Autodesk Fusion 360 part; units mm, degrees
sketch "Sketch1" plane through (0, 0, 0) normal (0, 0, 1) x (1, 0, 0)
  line L0 (30.2, 81.2805) -> (41.5, 81.2805)
  line L1 (41.5, 81.2805) -> (41.5, -5.4195)
  line L2 (41.5, -5.4195) -> (30.2, -5.4195)
  line L3 (30.2, -5.4195) -> (30.2, 81.2805)
  circle A0 centre (36.5, 3.0805) radius 1.5
  circle A1 centre (35.2, 72.7805) radius 1.5
  dimension "d1" = 1.3
  dimension "d2" = 69.7
  dimension "d3" = 3
  dimension "d4" = 3
  dimension "d5" = 5
  dimension "d6" = 5
  dimension "d7" = 8.5
  dimension "d8" = 8.5
extrude "Extrude1" add sketch "Sketch1" along normal blind 3
sketch "Sketch2" plane through (0, 0, 3) normal (0, 0, 1) x (-1, 0, 0)
  circle A0 centre (-36.5, -3.0805) radius 1.5
  circle A1 centre (-35.2, -72.7805) radius 1.5
  line L0 (-30.2, 5.4195) -> (-41.5, 5.4195)
  line L1 (-41.5, 5.4195) -> (-41.5, -81.2805)
  line L2 (-41.5, -81.2805) -> (-30.2, -81.2805)
  line L3 (-30.2, -81.2805) -> (-30.2, 5.4195)
  line L4 (-30.2, -53.1183) -> (-41.5, -53.1183)
  line L5 (-41.5, -53.1183) -> (-41.5, -31.956)
  line L6 (-41.5, -31.956) -> (-30.2, -31.956)
  line L7 (-30.2, -31.956) -> (-30.2, -53.1183)
extrude "Extrude2" add sketch "Sketch2" along normal blind 38.1 contours L1 L3 L4 L5 L6 L7
sketch "Sketch3" plane through (41.5, 0, 0) normal (1, 0, 0) x (0, 1, 0)
  line L0 (-5.4195, 0) -> (81.2805, 0)
  line L1 (81.2805, 0) -> (81.2805, 3)
  line L2 (81.2805, 3) -> (53.1183, 3)
  line L3 (53.1183, 3) -> (53.1183, 41.1)
  line L4 (53.1183, 41.1) -> (31.956, 41.1)
  line L5 (31.956, 41.1) -> (31.956, 3)
  line L6 (31.956, 3) -> (-5.4195, 3)
  line L7 (-5.4195, 3) -> (-5.4195, 0)
  line L8 (31.956, 34.75) -> (47, 34.75)
  line L9 (47, 34.75) -> (47, 31.575)
  line L10 (47, 31.575) -> (31.956, 31.575)
  line L11 (31.956, 31.575) -> (31.956, 34.75)
  line L12 (31.956, 12.525) -> (47, 12.525)
  line L13 (47, 12.525) -> (47, 9.35)
  line L14 (47, 9.35) -> (31.956, 9.35)
  line L15 (31.956, 9.35) -> (31.956, 12.525)
  dimension "d13" = 3.175
  dimension "d14" = 3.175
  dimension "d15" = 19.05
  dimension "d16" = 6.35
extrude "Extrude3" cut sketch "Sketch3" against normal blind 15 contours L5 L12 L13 L14 L15 | L5 L8 L9 L10 L11
sketch "Sketch4" plane through (0, 0, 41.1) normal (0, 0, 1) x (-1, 0, 0)
  line L0 (-30.2, -31.956) -> (-41.5, -31.956)
  line L1 (-41.5, -31.956) -> (-41.5, -53.1183)
  line L2 (-41.5, -53.1183) -> (-30.2, -53.1183)
  line L3 (-30.2, -53.1183) -> (-30.2, -31.956)
  circle A0 centre (-35.85, -34.956) radius 1.5
  circle A1 centre (-35.85, -42.956) radius 1.5
  dimension "d19" = 3
  dimension "d20" = 3
  dimension "d21" = 3
  dimension "d22" = 8
extrude "Extrude4" cut sketch "Sketch4" against normal blind 30 contours A0 | A1
Verification items for the finished model (mm, model axes). A direction names the side the tool comes from. Give positions to 0.01 mm unless a question says otherwise; leave off trailing zeros. Order: outer loops, then holes, each group sorted by start corner. A loop starts at its lowest first (then second) coordinate and runs counter-clockwise, first axis right, second up. Notation, with made-up numbers: (51.25, 37.5) -> (103.25, 37.5) arc R24 cw to (103.25, 48.5) -> close; hole circle Ø9 at (65.25, 60). An arc over 180 degrees is marked (long way). One line per item, written item: value.
(1) Tool access check on faces 1 (the face through (36, 31.956, 22)), 2 (the face through (41.5, 41, 16)), 3 (the face through (35.16, 36.29, 37.97)), 4 (the face through (36, 40, 9.35)). Record the directions out of +Z, -Z, +X, -X, +Y, -Y that give a thin tool (end or side, any length) a straight path to the whole face; none if there is none.
Final values:
face 1: +Z, +X, -X, -Y
face 2: +Z, -Z, +X, +Y, -Y
face 3: +Z
face 4: +X, -X, -Y
(2) Scan lines: line 1 along Y through (x, z) = (35.85, 19); line 2 along Z through (x, y) = (40, 38) (3 decimals); line 3 along Y through (x, z) = (36.5, 0.7). Record each from-to range of solid material in increasing order. Write a range as [from, to].
Final values:
line 1: [31.96, 33.46], [36.46, 41.46], [44.46, 53.12]
line 2: [0, 9.35], [12.525, 31.575], [34.75, 41.1]
line 3: [-5.42, 1.58], [4.58, 72.03], [73.53, 81.28]
(3) Sectioned sample at D-D on z = 21.5. Record the cut outline in (x, y).
Final values:
outline: (30.2, 31.96) -> (41.5, 31.96) -> (41.5, 53.12) -> (30.2, 53.12) -> close; hole circle Ø3 at (35.85, 34.96); hole circle Ø3 at (35.85, 42.96)
(4) Gauge pin test, flat ends, axial feed: pin 1 (4 mm diameter, centred on x = 35.5, z = 31, fed in from +Y); pin 2 (3.5 mm diameter, centred on x = 33.5, z = 11, fed in from -Y); pin 3 (5.5 mm diameter, centred on x = 36.5, y = 19, fed in from +Z). Record the tip position at first contact, or that the pin passes through.
Final values:
pin 1: y = 53.12
pin 2: y = 31.96
pin 3: z = 3
(5) Sectioned sample at C-C on z = 11.5. Record the cut outline in (x, y), then the cut area to 3 significant figures.
Final values:
outline: (30.2, 47) -> (41.5, 47) -> (41.5, 53.12) -> (30.2, 53.12) -> close
area: 69.1 mm^2
(6) Sectioned sample at A-A on y = 40. Record the cut outline in (x, z) (3 decimals).
Final values:
outline: (30.2, 0) -> (41.5, 0) -> (41.5, 9.35) -> (30.2, 9.35) -> close; (30.2, 12.525) -> (41.5, 12.525) -> (41.5, 31.575) -> (30.2, 31.575) -> close; (30.2, 34.75) -> (41.5, 34.75) -> (41.5, 41.1) -> (30.2, 41.1) -> close
(7) Draft check along Z on faces 5 (the face through (36, 39, 12.525)), 6 (the face through (35.16, 44.29, 22.18)), 7 (the face through (36, 47, 33)), 8 (the face through (36, 67, 3)). Enter one of: pulls with the +Z half, pulls with the -Z half, needs draft (parallel to the pull), parting line crosses it, or undercut.
Final values:
face 5: undercut
face 6: needs draft
face 7: undercut
face 8: pulls with the +Z half
